from build123d import *

# Parameters (mm, degrees)
SKETCH1_W                    = 20
SKETCH1_H                    = 26
BOSS_EXTRUDE1_DEPTH          = 1.5
BOSS_EXTRUDE1_DRAFT          = -5
SKETCH1_2_W                  = 20
SKETCH1_2_H                  = 26
BOSS_EXTRUDE2_DEPTH          = 3.5
BOSS_EXTRUDE2_TAPER          = 5
CUT_EXTRUDE1_DEPTH           = 3.5
CUT_EXTRUDE1_TAPER           = -5
CUT_EXTRUDE1_2_DEPTH         = 3.5
CUT_EXTRUDE1_2_TAPER         = -5
CUT_EXTRUDE1_3_DEPTH         = 3.5
CUT_EXTRUDE1_3_TAPER         = -5
CUT_EXTRUDE1_4_DEPTH         = 3.5
CUT_EXTRUDE1_4_TAPER         = -5
CUT_EXTRUDE3_DEPTH           = 17.770509989
CUT_EXTRUDE3_DEPTH_BACK      = 17.770509989
SKETCH5_5_R                  = 1.65
CUT_EXTRUDE4_START           = 3.5
SKETCH5_8_R                  = 0.75
CUT_EXTRUDE4_DEPTH           = 0.01
CUT_EXTRUDE5_START           = -1.5
SKETCH5_9_R                  = 1
CUT_EXTRUDE5_DEPTH           = 1
CUT_EXTRUDE5_DRAFT           = 30
CUT_EXTRUDE5_PROFILE_2_DEPTH = 1
CUT_EXTRUDE5_PROFILE_2_DRAFT = 30
SKETCH6_R                    = 3.5
CUT_EXTRUDE6_DEPTH           = 0.0001
SKETCH7_W                    = 3
SKETCH7_H                    = 0.56
SKETCH7_W_2                  = 2.5
BOSS_EXTRUDE3_DEPTH          = 2.1
SKETCH8_W                    = 1
SKETCH8_H                    = 0.56
BOSS_EXTRUDE4_DEPTH          = 18
FILLET1_R                    = 1


# Read off the part's stored shape, not the designer's step: Cut-Extrude1
with BuildPart() as part:
    # Sketch1 → Boss-Extrude1 (with draft: the straight prism first)
    with BuildSketch(Plane.XY):
        Rectangle(SKETCH1_W, SKETCH1_H)
    extrude(amount=-BOSS_EXTRUDE1_DEPTH)
    # Boss-Extrude1: the draft: its side faces are tilted about the plane it starts from
    boss_extrude1_sides = [part.faces().sort_by_distance(p)[0] for p in [
        (-10, 0, -0.75),
        (0, -13, -0.75),
        (10, 0, -0.75),
        (0, 13, -0.75),
    ]]
    draft(boss_extrude1_sides, Plane.XY, BOSS_EXTRUDE1_DRAFT)

    # Sketch1<2> → Boss-Extrude2 (add)
    with BuildSketch(Plane.XY):
        Rectangle(SKETCH1_2_W, SKETCH1_2_H)
    extrude(amount=BOSS_EXTRUDE2_DEPTH, taper=BOSS_EXTRUDE2_TAPER)

    # Cut-Extrude1 outline → Cut-Extrude1 (cut)
    with BuildSketch(Plane.XY):
        with BuildLine():
            Line((10, -1), (9.693789678, -1))
            ThreePointArc((9.693789678, -1), (8.693789678, -2), (9.693789678, -3))
            Line((9.693789678, -3), (10, -3))
            Line((10, -3), (10, -1))
        make_face()
    extrude(amount=CUT_EXTRUDE1_DEPTH, taper=CUT_EXTRUDE1_TAPER, mode=Mode.SUBTRACT)

    # Cut-Extrude1 2 outline → Cut-Extrude1 2 (cut)
    with BuildSketch(Plane.XY):
        with BuildLine():
            Line((-9.693789678, -1), (-10, -1))
            Line((-10, -1), (-10, -3))
            Line((-10, -3), (-9.693789678, -3))
            ThreePointArc((-9.693789678, -3), (-8.693789678, -2), (-9.693789678, -1))
        make_face()
    extrude(amount=CUT_EXTRUDE1_2_DEPTH, taper=CUT_EXTRUDE1_2_TAPER, mode=Mode.SUBTRACT)

    # Cut-Extrude1 3 outline → Cut-Extrude1 3 (cut)
    with BuildSketch(Plane.XY):
        with BuildLine():
            Line((-8.3, 9), (-10, 9))
            Line((-10, 9), (-10, 5))
            Line((-10, 5), (-8.3, 5))
            ThreePointArc((-8.3, 5), (-6.3, 7), (-8.3, 9))
        make_face()
    extrude(amount=CUT_EXTRUDE1_3_DEPTH, taper=CUT_EXTRUDE1_3_TAPER, mode=Mode.SUBTRACT)

    # Cut-Extrude1 4 outline → Cut-Extrude1 4 (cut)
    with BuildSketch(Plane.XY):
        with BuildLine():
            Line((10, 9), (8.3, 9))
            ThreePointArc((8.3, 9), (6.3, 7), (8.3, 5))
            Line((8.3, 5), (10, 5))
            Line((10, 5), (10, 9))
        make_face()
    extrude(amount=CUT_EXTRUDE1_4_DEPTH, taper=CUT_EXTRUDE1_4_TAPER, mode=Mode.SUBTRACT)

    # Sketch5<5> → Cut-Extrude3 (cut, two sides: drawn at the far end of the back side and taken through both)
    with BuildSketch(Plane.XY.offset(-CUT_EXTRUDE3_DEPTH_BACK)):
        with Locations((0, 7)):
            Circle(SKETCH5_5_R)
    extrude(amount=CUT_EXTRUDE3_DEPTH + CUT_EXTRUDE3_DEPTH_BACK, mode=Mode.SUBTRACT)

    # Sketch5<8> → Cut-Extrude4 (cut)
    with BuildSketch(Plane.XY.offset(CUT_EXTRUDE4_START)):
        with Locations((3.975, 7)):
            Circle(SKETCH5_8_R)
        with Locations((-3.975, 7)):
            Circle(SKETCH5_8_R)
        with Locations((0, -10.4)):
            Circle(SKETCH5_8_R)
        with BuildLine():
            Line((-6.1, 3.3), (6.1, 3.3))
            ThreePointArc((6.1, 3.3), (6.807106781, 3.007106781), (7.1, 2.3))
            Line((7.1, 2.3), (7.1, -6.3))
            ThreePointArc((7.1, -6.3), (6.807106781, -7.007106781), (6.1, -7.3))
            Line((6.1, -7.3), (-6.1, -7.3))
            ThreePointArc((-6.1, -7.3), (-6.807106781, -7.007106781), (-7.1, -6.3))
            Line((-7.1, -6.3), (-7.1, 2.3))
            ThreePointArc((-7.1, 2.3), (-6.807106781, 3.007106781), (-6.1, 3.3))
        make_face()
    extrude(amount=-CUT_EXTRUDE4_DEPTH, mode=Mode.SUBTRACT)


with BuildPart() as cut_extrude5_tool:
    # Sketch5<9> → Cut-Extrude5 (with draft: the straight prism first)
    with BuildSketch(Plane.XY.offset(CUT_EXTRUDE5_START)):
        with Locations((8.3, 7)):
            Circle(SKETCH5_9_R)
    extrude(amount=CUT_EXTRUDE5_DEPTH)
    # Cut-Extrude5: the draft: its side faces are tilted about the plane it starts from
    cut_extrude5_sides = [cut_extrude5_tool.faces().sort_by_distance(p)[0] for p in [
        (7.3, 7, -1),
    ]]
    draft(cut_extrude5_sides, Plane.XY.offset(CUT_EXTRUDE5_START), CUT_EXTRUDE5_DRAFT)


with BuildPart() as part_1:
    add(part.part)

    # Cut-Extrude5: cut by cut_extrude5_tool
    add(cut_extrude5_tool.part, mode=Mode.SUBTRACT)


with BuildPart() as cut_extrude5_profile_2_tool:
    # Sketch5<9> → Cut-Extrude5 profile 2 (with draft: the straight prism first)
    with BuildSketch(Plane.XY.offset(CUT_EXTRUDE5_START)):
        with Locations((-8.3, 7)):
            Circle(SKETCH5_9_R)
    extrude(amount=CUT_EXTRUDE5_PROFILE_2_DEPTH)
    # Cut-Extrude5 profile 2: the draft: its side faces are tilted about the plane it starts from
    cut_extrude5_profile_2_sides = [cut_extrude5_profile_2_tool.faces().sort_by_distance(p)[0] for p in [
        (-9.3, 7, -1),
    ]]
    draft(cut_extrude5_profile_2_sides, Plane.XY.offset(CUT_EXTRUDE5_START), CUT_EXTRUDE5_PROFILE_2_DRAFT)


with BuildPart() as part_2:
    add(part_1.part)

    # Cut-Extrude5 profile 2: cut by cut_extrude5_profile_2_tool
    add(cut_extrude5_profile_2_tool.part, mode=Mode.SUBTRACT)

    # Sketch6 → Cut-Extrude6 (cut)
    with BuildSketch(Plane(origin=(0, 0, -1.5), x_dir=(-1, 0, 0), z_dir=(0, 0, -1))):
        with BuildLine():
            Line((-5.427124344, 11.5), (5.427124344, 11.5))
            ThreePointArc((5.427124344, 11.5), (6.75, 12), (8.072875656, 11.5))
            Line((8.072875656, 11.5), (9, 10.578427125))
            Line((9, 10.578427125), (9, 8.5))
            ThreePointArc((9, 8.5), (7.3, 7), (9, 5.5))
            Line((9, 5.5), (9, -9))
            Line((9, -9), (-9, -9))
            Line((-9, -9), (-9, 5.5))
            ThreePointArc((-9, 5.5), (-7.3, 7), (-9, 8.5))
            Line((-9, 8.5), (-9, 10.578427125))
            Line((-9, 10.578427125), (-8.164213562, 11.414213562))
            ThreePointArc((-8.164213562, 11.414213562), (-6.812653663, 11.999018389), (-5.427124344, 11.5))
        make_face()
        with Locations((0, 7)):
            Circle(SKETCH6_R, mode=Mode.SUBTRACT)
    extrude(amount=-CUT_EXTRUDE6_DEPTH, mode=Mode.SUBTRACT)

    # Sketch7 → Boss-Extrude3 (add)
    with BuildSketch(Plane(origin=(0, -12.800597138, 0.447962854), x_dir=(-1, 0, 0), z_dir=(0, -0.9993882205697596, 0.034974055904479696))):
        with Locations((0, 0.026094538)):
            Rectangle(SKETCH7_W, SKETCH7_H)
        with Locations((-5.31, 0.026094538)):
            Rectangle(SKETCH7_W_2, SKETCH7_H)
        with Locations((5.31, 0.026094538)):
            Rectangle(SKETCH7_W_2, SKETCH7_H)
    extrude(amount=BOSS_EXTRUDE3_DEPTH)

    # Sketch8 → Boss-Extrude4 (add)
    with BuildSketch(Plane(origin=(0, -14.899312401, 0.521408372), x_dir=(1, 0, 0), z_dir=(0, -0.9993882205697596, 0.03497405590447946))):
        with Locations((5.31, -0.026094538)):
            Rectangle(SKETCH8_W, SKETCH8_H)
        with Locations((0, -0.026094538)):
            Rectangle(SKETCH8_W, SKETCH8_H)
        with Locations((-5.31, -0.026094538)):
            Rectangle(SKETCH8_W, SKETCH8_H)
    extrude(amount=BOSS_EXTRUDE4_DEPTH)

    # Fillet1
    # the kernel refuses this fillet: 1 mm, written as the material it adds along each edge
    with BuildSketch(Plane(origin=(4.81, -14.910017769, 0.215501096), x_dir=(-1, 0, 0), z_dir=(0, 0.03497405590447946, 0.9993882205697596)), Plane(origin=(5.81, -14.890432297, 0.7751585), x_dir=(1, 0, 0), z_dir=(0, -0.03497405590447946, -0.9993882205697596)), Plane(origin=(-5.81, -14.910017769, 0.215501096), x_dir=(-1, 0, 0), z_dir=(0, 0.03497405590447946, 0.9993882205697596)), Plane(origin=(-4.81, -14.890432297, 0.7751585), x_dir=(1, 0, 0), z_dir=(0, -0.03497405590447946, -0.9993882205697596))) as fillet1_piece_1:
        with BuildLine():
            CenterArc((1, 0.968245837), FILLET1_R, 180, 75.522487814)
            Line((0, 0.968245837), (-0.02, 0.968245837))
            Line((-0.02, 0.968245837), (-0.02, 0))
            Line((-0.02, 0), (0, -0.02))
            ThreePointArc((0, -0.02), (0.375, -0.02), (0.745, -0.019364917))
            Line((0.745, -0.019364917), (0.75, 0))
        make_face()
    extrude(amount=0.56)
    with BuildSketch(Plane(origin=(0.5, -14.910017769, 0.215501096), x_dir=(1, 0, 0), z_dir=(0, 0.03497405590447946, 0.9993882205697596)), Plane(origin=(-0.5, -14.890432297, 0.7751585), x_dir=(-1, 0, 0), z_dir=(0, -0.03497405590447946, -0.9993882205697596))) as fillet1_piece_2:
        with BuildLine():
            CenterArc((FILLET1_R, -FILLET1_R), FILLET1_R, 90, 90)
            Line((0, -FILLET1_R), (-FILLET1_R * 0.02, -FILLET1_R))
            Line((-FILLET1_R * 0.02, -FILLET1_R), (-FILLET1_R * 0.02, FILLET1_R * 0.02))
            Line((-FILLET1_R * 0.02, FILLET1_R * 0.02), (FILLET1_R, FILLET1_R * 0.02))
            Line((FILLET1_R, FILLET1_R * 0.02), (FILLET1_R, 0))
        make_face()
    extrude(amount=0.56)


solid = part_2.part
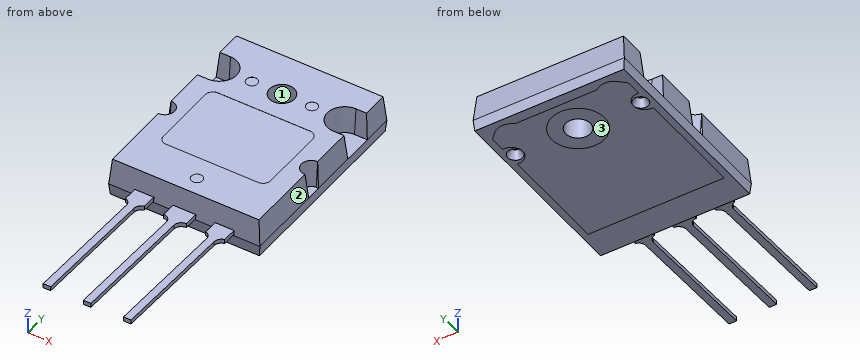
CAD build for the part. Positions are in the model's coordinates, mm. Face numbers are marked on the shaded views. Give positions to 0.01 mm unless a question says otherwise; leave off trailing zeros. Write each loop counter-clockwise with the first axis right and the second up, starting at its lowest first coordinate (ties: lowest second). Pieces come first, ordered by that corner, then holes. Notation, with made-up numbers: (58.25, 82) - (71.25, 82) arc R29 cw to (71.25, 121) - close; hole circle Ø9 at (11, 72). An arc over 180 degrees is marked (long way). Answer as CSV lines item,"result".
Q1. Drill centre lines: line 1 (X direction, y = 7, z = 2.25); line 2 (Y direction, x = 7.75, z = 0.2); line 3 (Y direction, x = 7, z = 1.8). Where is each one in solid material? Low to high. Write a range as from..to.
Result set:
line 1,"-6.1..-1.65, 1.65..6.1"
line 2,"-12.98..5.06, 8.94..12.98"
line 3,"-12.84..5.28, 8.72..12.84"
Q2. Flat gauge pins, fed straight in: pin 1 Ø1.2 at (x, y) = (4, 7) entering from +Z; pin 2 Ø1.5 at (y, z) = (5, 2) entering from +X; pin 3 Ø0.7 at (y, z) = (-13.5, 0.5) entering from -X; pin 4 Ø2 at (y, z) = (-14.5, 2) entering from -X. Where does each tip first touch, or does it go through?
Result set:
pin 1,"z = 3.49"
pin 2,"x = 9.89"
pin 3,"x = -6.56"
pin 4,"through"
Q3. Band-saw the part on C-C (y = -26). Give the cut face in (x, z).
Result set:
outline,"(-5.81, 0.6) - (-4.81, 0.6) - (-4.81, 1.16) - (-5.81, 1.16) - close; (-0.5, 0.6) - (0.5, 0.6) - (0.5, 1.16) - (-0.5, 1.16) - close; (4.81, 0.6) - (5.81, 0.6) - (5.81, 1.16) - (4.81, 1.16) - close"
Q4. Pull direction X, two halves, no side cores. Call the marked faces 1, 2 and 3: released by +X, released by -X, zero draft, split by the parting line, or undercut.
Result set:
face 1,"undercut"
face 2,"released by +X"
face 3,"zero draft"
